Work out the finished part from the listing and answer in its coordinate system (mm). Coordinates: 2 decimals unless noted, no trailing zeros. Order: outer loops, then holes, each group sorted by start corner. A loop starts at its lowest first (then second) coordinate and runs counter-clockwise, first axis right, second up. Notation, with made-up numbers: M 43.5,-15 L 65.5,-15 A24 ccw 65.5,4 Z; hole C 63.25,-36.5 d6. An arc over 180 degrees is marked long. Write item = value, one per line. Start each with the question number.
Q1. Straight lines are drawn through the part: line 1 along X through (y, z) = (-2, 3); line 2 along X through (y, z) = (2.75, 4.75); line 3 along Y through (x, z) = (-44, 0.6). For each, find the intervals that lie inside material, in ascending order.
Q2. Find section A-A on z = 1.15. Give the vertices of the cut face in (x, y).
Q3. Each of these flat-tipped pins is pushed along its axis until it touches: P1, Ø2.5, axis at x = 36, z = 1.5, coming from the +Y side; P2, Ø1.5, axis at x = -21.5, z = 3, coming from the -Y side; P3, Ø1.2, axis at y = 2.5, z = 2, coming from the +X side. Where does it stop, or does it pass through?
Q4. Find section B-B on x = 34. Give the vertices of the cut face in (y, z), and give its area (3 significant figures).
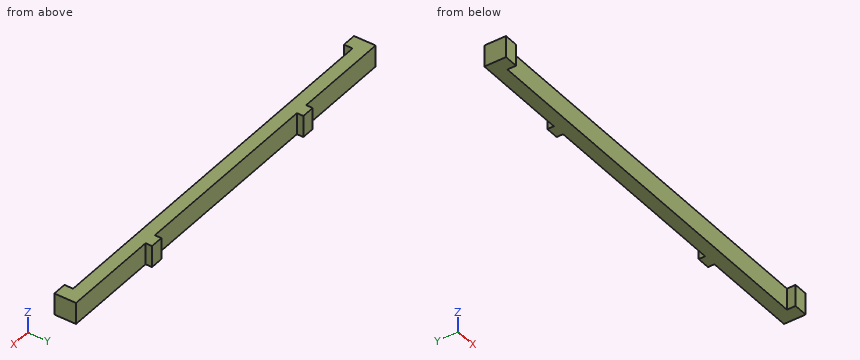
```python
from build123d import *

# Parameters (mm, degrees)
F0_W     = 3
F0_H     = 1.5
F1_DEPTH = 5


with BuildPart() as f1:
    # F0 (on Top) → F1 (new body)
    with BuildSketch(Plane.XY):
        Polygon((-45.25, -3.5), (-45.25, -1.5), (-45.25, 1.5), (-48.5, 1.5), (-48.5, -3.5), align=None)
        with Locations((-24.5, 2.25)):
            Rectangle(F0_W, F0_H)
        Polygon((-45.25, -1.5), (45.25, -1.5), (45.25, 1.5), (26, 1.5), (23, 1.5), (-23, 1.5), (-26, 1.5), (-45.25, 1.5), align=None)
        with Locations((24.5, 2.25)):
            Rectangle(F0_W, F0_H)
        Polygon((45.25, 1.5), (45.25, -1.5), (45.25, -3.5), (48.5, -3.5), (48.5, 1.5), align=None)
    extrude(amount=F1_DEPTH)


solid = f1.part
```
Findings below:
q1.line_1 = -48.5 to -45.25, 45.25 to 48.5
q1.line_2 = -26 to -23, 23 to 26
q1.line_3 = -1.5 to 1.5
q2.outline = M -48.5,-3.5 L -45.25,-3.5 L -45.25,-1.5 L 45.25,-1.5 L 45.25,-3.5 L 48.5,-3.5 L 48.5,1.5 L 26,1.5 L 26,3 L 23,3 L 23,1.5 L -23,1.5 L -23,3 L -26,3 L -26,1.5 L -48.5,1.5 Z
q3.P1 = 1.5
q3.P2 = -1.5
q3.P3 = 26
q4.outline = M -1.5,0 L 1.5,0 L 1.5,5 L -1.5,5 Z
q4.area = 15.0 mm^2
